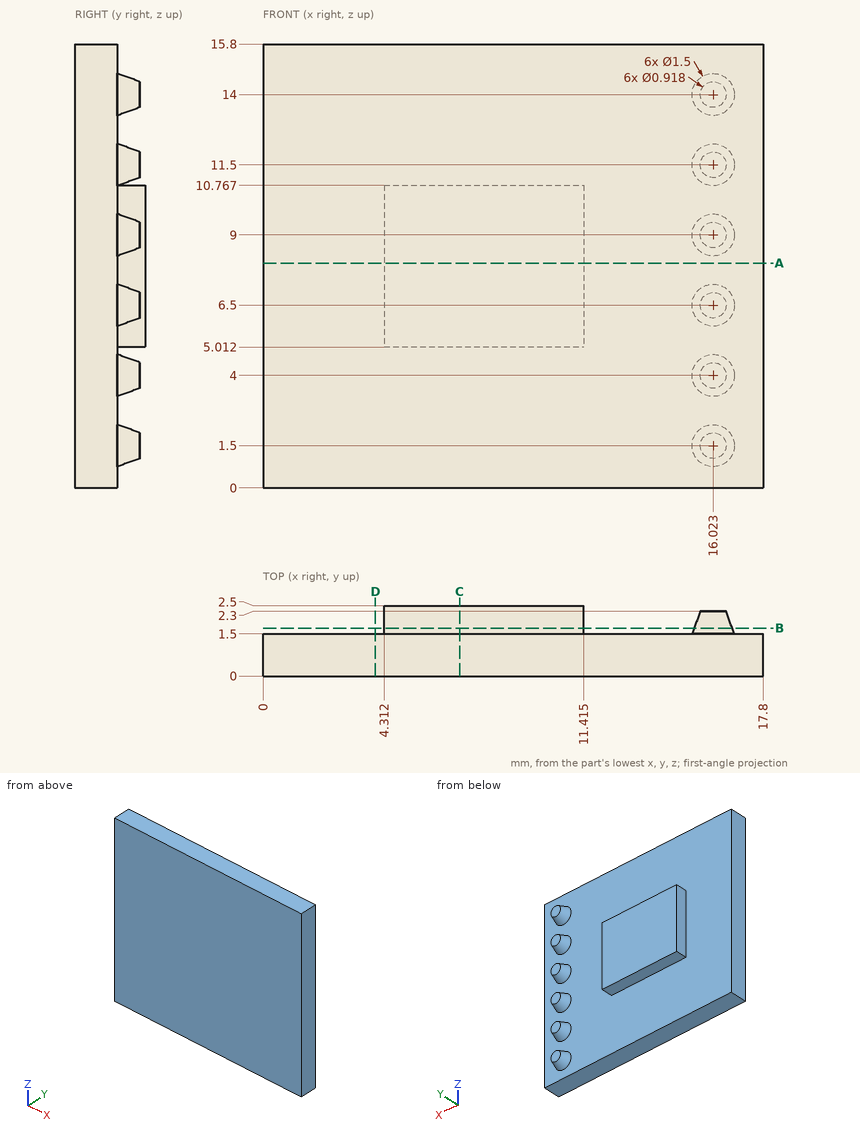
Check sheet for the drawn part. Datum: minimum x, y, z corner. Units: mm. Give positions to 0.01 mm unless a question says otherwise; leave off trailing zeros. Loops run counter-clockwise (first coordinate to the right, second up) from the corner with the lowest first, then second, coordinate; pieces in that order, holes last.
1) Thickness scan on line 1 along Y through (x, z) = (6.25, 12.5); line 2 along Z through (x, y) = (8.5, 2.05); line 3 along Y through (x, z) = (15.75, 8.75). Record the ranges inside material, lowest first.
2) Sectioned sample at B-B, the plane y = 1.7. Enter the section's corners in (x, z) (1 decimal).
3) Sectioned sample at A-A, the plane z = 8. Enter the section's corners in (x, y) (1 decimal).
4) Sectioned sample at D-D, the plane x = 4. Enter the section's corners in (y, z).
5) Depth check by flat-ended pin: pin 1 Ø1 at (y, z) = (1.5, 7) entering from -X; pin 2 Ø0.5 at (x, z) = (16, 6.5) entering from +Y; pin 3 Ø0.5 at (y, z) = (2, 7) entering from +X; pin 4 Ø0.8 at (x, y) = (8.5, 2) entering from -Z. Enter the tip coordinate at first touch or a pass-through.
6) Sectioned sample at C-C, the plane x = 7. Enter the section's corners in (y, z).
Answers:
1. line 1: y = 0 to 1.5
1. line 2: z = 5.01 to 10.77
1. line 3: y = 0 to 2.3
2. outline: (4.3, 5) - (11.4, 5) - (11.4, 10.8) - (4.3, 10.8) - close; circle Ø1.4 at (16, 1.5); circle Ø1.4 at (16, 4); circle Ø1.4 at (16, 6.5); circle Ø1.4 at (16, 9); circle Ø1.4 at (16, 11.5); circle Ø1.4 at (16, 14)
3. outline: (0, 0) - (17.8, 0) - (17.8, 1.5) - (11.4, 1.5) - (11.4, 2.5) - (4.3, 2.5) - (4.3, 1.5) - (0, 1.5) - close
4. outline: (0, 0) - (1.5, 0) - (1.5, 15.8) - (0, 15.8) - close
5. pin 1: stops at x = 0
5. pin 2: stops at y = 2.3
5. pin 3: stops at x = 16.57
5. pin 4: stops at z = 5.01
6. outline: (0, 0) - (1.5, 0) - (1.5, 5.01) - (2.5, 5.01) - (2.5, 10.77) - (1.5, 10.77) - (1.5, 15.8) - (0, 15.8) - close
